Design review of the part shown in the three views and the two pictorial views. Dimensions are in mm from the part's minimum x, y and z. A direction names the side the tool comes from. Give positions to 0.01 mm unless a question says otherwise; leave off trailing zeros. Order: outer loops, then holes, each group sorted by start corner. A loop starts at its lowest first (then second) coordinate and runs counter-clockwise, first axis right, second up. Notation, with made-up numbers: M 29.5,55.5 L 40.5,55.5 A21 cw 40.5,67.5 Z; hole C 64,-3.75 d9. An arc over 180 degrees is marked long. Answer as a JSON object with one key per item and string values.
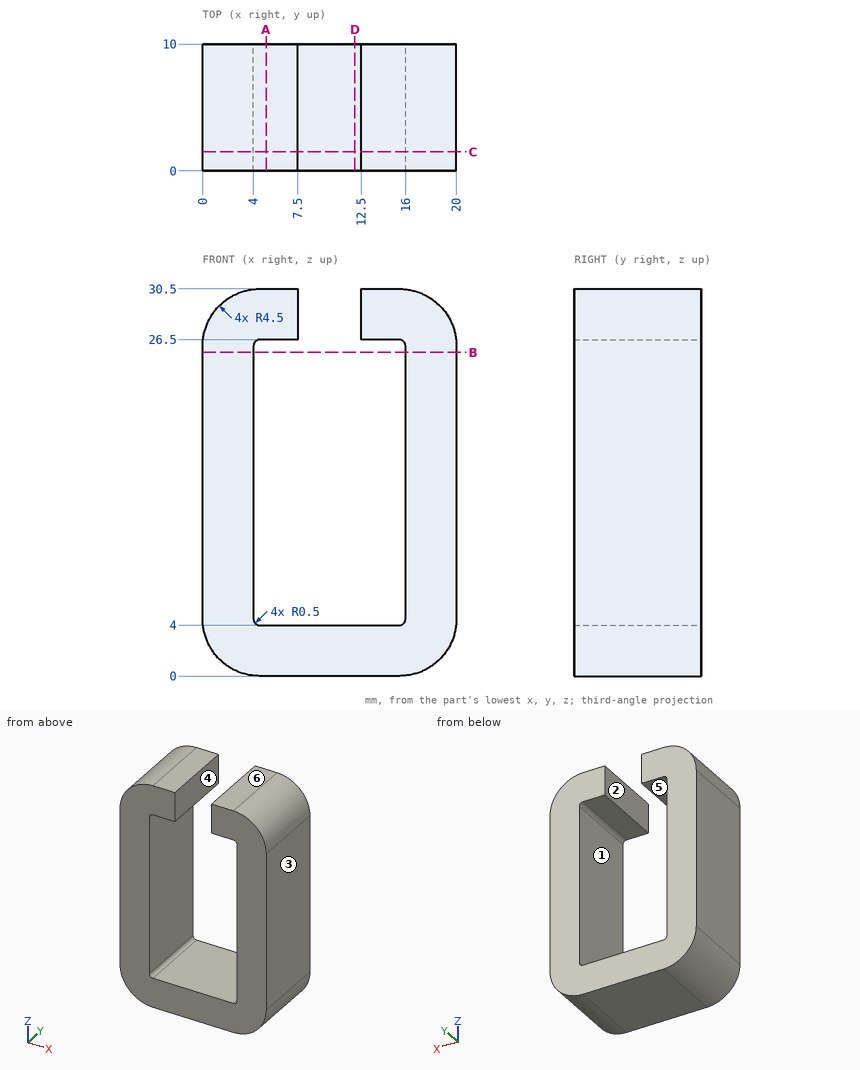
(1) Draft analysis for pull direction Z (two halves, no side actions). For the marked faces 4, 5 and 6, state which applies: +Z half, -Z half, draft (parallel to the pull), parting line (faces both ways), or undercut.
Checked values:
{"face 4": "draft", "face 5": "undercut", "face 6": "+Z half"}
(2) We need section A-A (x = 5). Write out the cut boundary in (y, z), plus the area to 3 significant figures.
Checked values:
{"outline": "M 0,0 L 10,0 L 10,4 L 0,4 Z; M 0,26.5 L 10,26.5 L 10,30.5 L 0,30.5 Z", "area": "80.0 mm^2"}
(3) To check wall thickness, follow L1, parallel to X at y = 7.25, z = 6; L2, parallel to Z at x = 6.25, y = 9.5; L3, parallel to Z at x = 9.75, y = 1. State the ranges of each line that lie inside material, in increasing order. Write a range as from..to.
Checked values:
{"L1": "x = 0..4, 16..20", "L2": "z = 0..4, 26.5..30.5", "L3": "z = 0..4"}
(4) We need section C-C (y = 1.5). Write out the cut boundary in (x, z).
Checked values:
{"outline": "M 0,4.5 A4.5 ccw 4.5,0 L 15.5,0 A4.5 ccw 20,4.5 L 20,26 A4.5 ccw 15.5,30.5 L 12.5,30.5 L 12.5,26.5 L 15.5,26.5 A0.5 cw 16,26 L 16,4.5 A0.5 cw 15.5,4 L 4.5,4 A0.5 cw 4,4.5 L 4,26 A0.5 cw 4.5,26.5 L 7.5,26.5 L 7.5,30.5 L 4.5,30.5 A4.5 ccw 0,26 Z"}
(5) We need section D-D (x = 12). Write out the cut boundary in (y, z).
Checked values:
{"outline": "M 0,0 L 10,0 L 10,4 L 0,4 Z"}
(6) Insertion check: pin 1 (10 mm diameter, centred on x = 12, z = 19.5, fed in from -Y); pin 2 (4.5 mm diameter, centred on y = 5, z = 29, fed in from +X); pin 3 (3 mm diameter, centred on y = 5.5, z = 28, fed in from -X). Each pin has a flat end and moves straight along its axis. Give the tip position at first contact, or say it passes through.
Checked values:
{"pin 1": "stops at y = 0", "pin 2": "stops at x = 19.94", "pin 3": "stops at x = 0.03"}
(7) We need section B-B (z = 25.5). Write out the cut boundary in (x, y).
Checked values:
{"outline": "M 0,0 L 4,0 L 4,10 L 0,10 Z; M 16,0 L 20,0 L 20,10 L 16,10 Z"}
(8) Tool access review of the marked faces 1, 2 and 3: name each direction out of +Z, -Z, +X, -X, +Y, -Y from which nothing blocks a thin tool from reaching the whole face with its end or side.
Checked values:
{"face 1": "+Y, -Y", "face 2": "+Z, +Y, -Y", "face 3": "+Z, -Z, +X, +Y, -Y"}
